Design review of the part built by this model. Coordinates are the model's own, in mm. Coordinates: 2 decimals unless noted, no trailing zeros. Loops run counter-clockwise (first coordinate to the right, second up) from the corner with the lowest first, then second, coordinate; pieces in that order, holes last. Notation, with made-up numbers: (-11.75, 8) -> (17.25, 8) arc R9 cw to (17.25, 22) -> close; hole circle Ø10 at (-37, -37). An arc over 180 degrees is marked (long way). One line per item, written item: value. Start each with the question number.
1. Add section B-B on z = -23.5. Write out the cut boundary in (x, y), plus the area to 3 significant figures.
2. Add section A-A on x = -35.5. Write out the cut boundary in (y, z).
3. For probe 1 along X at (y, z) = (-0.7, 11.24); probe 2 along X at (y, z) = (-0.45, -27.76); probe 3 along X at (y, z) = (-0.3, 16.74), list the stretches that pass through material, from the lowest coordinate up.
4. Add section C-C on z = -42. Write out the cut boundary in (x, y).
5. Insertion check: pin 1 (0.5 mm diameter, centred on y = -0.5, z = -40, fed in from -X); pin 2 (8 mm diameter, centred on x = -44.5, z = 3.5, fed in from +Y); pin 3 (1.1 mm diameter, centred on y = -0.5, z = -18, fed in from +X). Each pin has a flat end and moves straight along its axis. Give the tip position at first contact, or say it passes through.
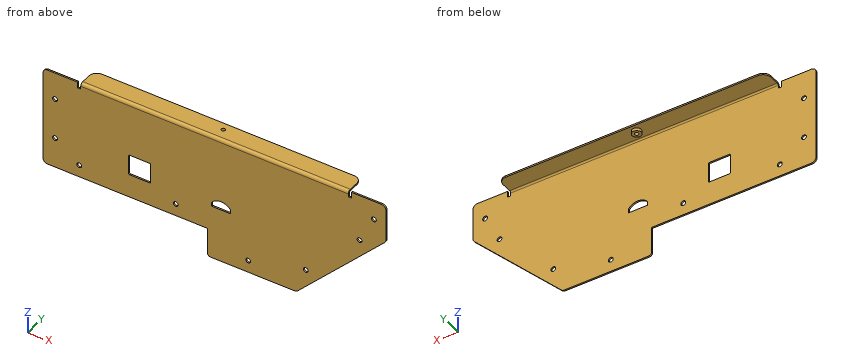
```python
from build123d import *

# Parameters (mm, degrees)
SKETCH_1_R                        = 1.6
SM_BASE_FLANGE_1_DEPTH            = 1
SM_EDGE_FLANGE_1_STRIP_W          = 6
SM_EDGE_FLANGE_1_STRIP_H          = 1
SM_EDGE_FLANGE_1_STRIP_CUT_DEPTH  = 177.34
SM_EDGE_FLANGE_1_RELIEF_W         = 8
SM_EDGE_FLANGE_1_RELIEF_H         = 2
SM_EDGE_FLANGE_1_RELIEF_CUT_DEPTH = 1
SM_EDGE_FLANGE_1_DEPTH            = 177.34
SM_EDGE_FLANGE_1_FLAT_DEPTH       = 1
SKETCH_5_R                        = 3
EXTRUDE_1_DEPTH                   = 2
HOLE_WIZARD_M3_1_D                = 2.5


# Sheet-metal steps are written as plain solids
with BuildPart() as part:
    # Sketch 1 → 基体-法兰1 (new body)
    with BuildSketch(Plane(origin=(0, 0, 0), x_dir=(1, 0, 0), z_dir=(0, 1, 0))):
        with BuildLine():
            Line((-113.67, 32.76), (-113.67, -26.24))
            ThreePointArc((-113.67, -26.24), (-112.791320344, -28.361320344), (-110.67, -29.24))
            Line((-110.67, -29.24), (110.67, -29.24))
            ThreePointArc((110.67, -29.24), (112.791320344, -28.361320344), (113.67, -26.24))
            Line((113.67, -26.24), (113.67, -5.882640687))
            ThreePointArc((113.67, -5.882640687), (113.441638598, -4.73459039), (112.791320344, -3.761320344))
            Line((112.791320344, -3.761320344), (55.148679656, 53.881320344))
            ThreePointArc((55.148679656, 53.881320344), (54.17540961, 54.531638598), (53.027359313, 54.76))
            Line((53.027359313, 54.76), (-2.67, 54.76))
            ThreePointArc((-2.67, 54.76), (-4.084213562, 54.174213562), (-4.67, 52.76))
            Line((-4.67, 52.76), (-4.67, 35.76))
            Line((-4.67, 35.76), (-110.67, 35.76))
            ThreePointArc((-110.67, 35.76), (-112.791320344, 34.881320344), (-113.67, 32.76))
        make_face()
        with Locations(Location((-105.67, -11.24, 0), (0, 0, 270))):
            Circle(SKETCH_1_R, mode=Mode.SUBTRACT)
        with Locations(Location((-105.67, 15.76, 0), (0, 0, 270))):
            Circle(SKETCH_1_R, mode=Mode.SUBTRACT)
        with Locations(Location((-89.67, 27.76, 0), (0, 0, 270))):
            Circle(SKETCH_1_R, mode=Mode.SUBTRACT)
        with Locations(Location((-25.67, 27.76, 0), (0, 0, 270))):
            Circle(SKETCH_1_R, mode=Mode.SUBTRACT)
        with Locations(Location((22.33, 46.76, 0), (0, 0, 270))):
            Circle(SKETCH_1_R, mode=Mode.SUBTRACT)
        with Locations(Location((60.516291501, 37.2, 0), (0, 0, 270))):
            Circle(SKETCH_1_R, mode=Mode.SUBTRACT)
        with Locations(Location((96.116291501, 1.6, 0), (0, 0, 270))):
            Circle(SKETCH_1_R, mode=Mode.SUBTRACT)
        with Locations(Location((105.67, -16.74, 0), (0, 0, 270))):
            Circle(SKETCH_1_R, mode=Mode.SUBTRACT)
        with BuildLine():
            Line((10.63, 19.26), (-1.87, 19.26))
            Line((-1.87, 19.26), (-1.87, 16.56))
            ThreePointArc((-1.87, 16.56), (4.38, 13.553746089), (10.63, 16.56))
            Line((10.63, 16.56), (10.63, 19.26))
        make_face(mode=Mode.SUBTRACT)
        with BuildLine():
            Line((-42.37, 19.86), (-42.37, 7.36))
            ThreePointArc((-42.37, 7.36), (-42.516446609, 7.006446609), (-42.87, 6.86))
            Line((-42.87, 6.86), (-56.37, 6.86))
            ThreePointArc((-56.37, 6.86), (-56.723553391, 7.006446609), (-56.87, 7.36))
            Line((-56.87, 7.36), (-56.87, 19.86))
            ThreePointArc((-56.87, 19.86), (-56.723553391, 20.213553391), (-56.37, 20.36))
            Line((-56.37, 20.36), (-42.87, 20.36))
            ThreePointArc((-42.87, 20.36), (-42.516446609, 20.213553391), (-42.37, 19.86))
        make_face(mode=Mode.SUBTRACT)
    extrude(amount=-SM_BASE_FLANGE_1_DEPTH)

    # 边线-法兰1 strip (across the edge) → 边线-法兰1 strip cut (cut)
    with BuildSketch(Plane(origin=(-88.67, 0, 29.24), x_dir=(0, 0, -1), z_dir=(1, 0, 0))):
        with Locations((-1, -0.5)):
            Rectangle(SM_EDGE_FLANGE_1_STRIP_W, SM_EDGE_FLANGE_1_STRIP_H)
    extrude(amount=SM_EDGE_FLANGE_1_STRIP_CUT_DEPTH, mode=Mode.SUBTRACT)

    # 边线-法兰1 relief (on the sheet) → 边线-法兰1 relief cut (cut)
    with BuildSketch(Plane(origin=(-88.67, 0, 27.24), x_dir=(0, 0, -1), z_dir=(0, 1, 0))):
        with Locations((-2, 1)):
            Rectangle(SM_EDGE_FLANGE_1_RELIEF_W, SM_EDGE_FLANGE_1_RELIEF_H)
        with Locations((-2, -178.34)):
            Rectangle(SM_EDGE_FLANGE_1_RELIEF_W, SM_EDGE_FLANGE_1_RELIEF_H)
    extrude(amount=-SM_EDGE_FLANGE_1_RELIEF_CUT_DEPTH, mode=Mode.SUBTRACT)

    # 边线-法兰1 bend section (across the edge) → 边线-法兰1 (add)
    with BuildSketch(Plane(origin=(-88.67, 0, 29.24), x_dir=(0, 0, -1), z_dir=(1, 0, 0))):
        with BuildLine():
            Line((0, 1), (1, 1))
            ThreePointArc((1, 1), (1.292893219, 0.292893219), (2, 0))
            Line((2, 0), (2, -1))
            ThreePointArc((2, -1), (0.585786438, -0.414213562), (0, 1))
        make_face()
    extrude(amount=SM_EDGE_FLANGE_1_DEPTH)

    # 边线-法兰1 profile (on flange) → 边线-法兰1 flat (add)
    with BuildSketch(Plane.XY.offset(29.24)):
        with BuildLine():
            Line((-88.67, 1), (88.67, 1))
            Line((88.67, 1), (88.67, 7.5))
            ThreePointArc((88.67, 7.5), (87.205533906, 11.035533906), (83.67, 12.5))
            Line((83.67, 12.5), (-83.67, 12.5))
            ThreePointArc((-83.67, 12.5), (-87.205533906, 11.035533906), (-88.67, 7.5))
            Line((-88.67, 7.5), (-88.67, 1))
        make_face()
    extrude(amount=-SM_EDGE_FLANGE_1_FLAT_DEPTH)

    # 草图5 → 凸台-拉伸1 (add)
    with BuildSketch(Plane(origin=(0, 0, 28.24), x_dir=(-1, 0, 0), z_dir=(0, 0, -1))):
        with Locations((-0.17, 7.5)):
            Circle(SKETCH_5_R)
    extrude(amount=EXTRUDE_1_DEPTH)

    # M3 螺纹孔1 (through all)
    with Locations(Plane(origin=(0, 0, 26.24), x_dir=(-1, 0, 0), z_dir=(0, 0, -1))):
        with Locations((-0.17, 7.5)):
            Hole(HOLE_WIZARD_M3_1_D / 2)


solid = part.part
```
Worked answers:
1. outline: (-113.67, -1) -> (85.53, -1) -> (85.53, 0) -> (-113.67, 0) -> close
1. area: 199 mm²
2. outline: (-1, -35.76) -> (0, -35.76) -> (0, 27.24) arc R1 cw to (1, 28.24) -> (12.5, 28.24) -> (12.5, 29.24) -> (1, 29.24) arc R2 ccw to (-1, 27.24) -> close
3. probe 1: x = -113.67 to -107.27, -104.07 to 113.67
3. probe 2: x = -113.67 to -91.27, -88.07 to -27.27, -24.07 to 81.27
3. probe 3: x = -113.67 to 104.07, 107.27 to 113.67
4. outline: (-4.67, -1) -> (67.03, -1) -> (67.03, 0) -> (-4.67, 0) -> close
5. pin 1: stops at x = -4.67
5. pin 2: stops at y = 0
5. pin 3: stops at x = 91.58
